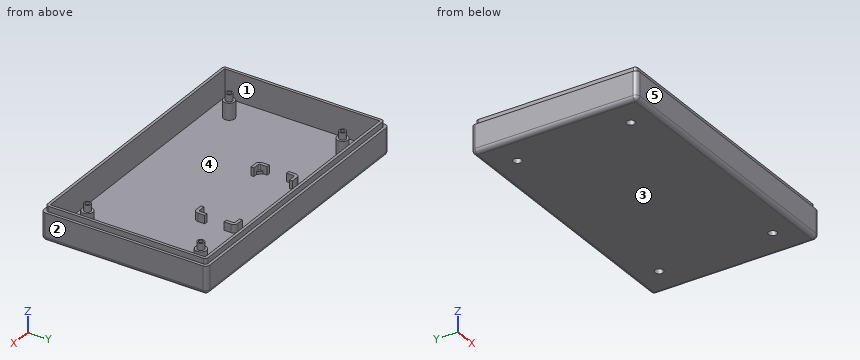
from build123d import *

# Parameters (mm, degrees)
SKETCH_1_W                  = 100
SKETCH_1_H                  = 60
EXTRUDE_1_DEPTH             = 2
SKETCH_2_W                  = 96
SKETCH_2_H                  = 56
EXTRUDE_2_DEPTH             = 10
SKETCH_3_W                  = 100
SKETCH_3_H                  = 60
SKETCH_3_W_2                = 98
SKETCH_3_H_2                = 58
CUT_EXTRUDE_1_DEPTH         = 2
EXTRUDE_3_DEPTH             = 3
EXTRUDE_4_DEPTH             = 1
FILLET_1_R                  = 0.5
FILLET_2_R                  = 1.5
SKETCH_6_R                  = 2
EXTRUDE_5_DEPTH             = 6
SKETCH_7_R                  = 1.2
EXTRUDE_6_DEPTH             = 2.5
SKETCH_8_R                  = 0.75
CUT_EXTRUDE_2_DEPTH         = 12.5
FILLET_3_R                  = 1.5
FILLET_4_R                  = 1.5
FILLET_5_R                  = 1
SKETCH_9_R                  = 1.5
CUT_EXTRUDE_3_DEPTH         = 7
PATTERN_LINEAR_1_COUNT      = 2
PATTERN_LINEAR_1_PITCH      = 78
PATTERN_LINEAR_1_COUNT_DIR2 = 2
PATTERN_LINEAR_1_PITCH_DIR2 = 41


with BuildPart() as part:
    # 草图1 → 凸台-拉伸1 (new body)
    with BuildSketch(Plane.XY):
        Rectangle(SKETCH_1_W, SKETCH_1_H)
    extrude(amount=EXTRUDE_1_DEPTH)

    # 草图2 → 凸台-拉伸2 (add)
    with BuildSketch(Plane.XY.offset(2)):
        Polygon((-47, 30), (-50, 30), (-50, 27), (-50, -27), (-50, -30), (-47, -30), (47, -30), (50, -30), (50, -27), (50, 27), (50, 30), (47, 30), align=None)
        Rectangle(SKETCH_2_W, SKETCH_2_H, mode=Mode.SUBTRACT)
    extrude(amount=EXTRUDE_2_DEPTH)

    # 草图3 → 切除-拉伸1 (cut)
    with BuildSketch(Plane.XY.offset(12)):
        Rectangle(SKETCH_3_W, SKETCH_3_H)
        Rectangle(SKETCH_3_W_2, SKETCH_3_H_2, mode=Mode.SUBTRACT)
    extrude(amount=-CUT_EXTRUDE_1_DEPTH, mode=Mode.SUBTRACT)

    # 草图4 → 凸台-拉伸3 (add)
    with BuildSketch(Plane.XY.offset(2)):
        Polygon((-16.61, 17.9), (-13.75, 17.9), (-13.75, 18.95), (-17.75, 18.95), (-17.75, 14.95), (-16.61, 14.95), align=None)
        Polygon((-16.61, 5), (-13.75, 5), (-13.75, 3.95), (-17.75, 3.95), (-17.75, 7.95), (-16.61, 7.95), align=None)
        Polygon((16.61, 17.9), (16.61, 14.95), (17.75, 14.95), (17.75, 18.95), (13.75, 18.95), (13.75, 17.9), align=None)
        Polygon((17.75, 3.95), (13.75, 3.95), (13.75, 5), (16.61, 5), (16.61, 7.95), (17.75, 7.95), align=None)
    extrude(amount=EXTRUDE_3_DEPTH)

    # 草图5 → 凸台-拉伸4 (add)
    with BuildSketch(Plane.XY.offset(2)):
        Polygon((-16.61, 17.9), (-15.11, 17.9), (-16.61, 16.4), align=None)
        Polygon((16.61, 17.9), (15.11, 17.9), (16.61, 16.4), align=None)
        Polygon((16.61, 5), (16.61, 6.5), (15.11, 5), align=None)
        Polygon((-16.61, 5), (-15.11, 5), (-16.61, 6.5), align=None)
    extrude(amount=EXTRUDE_4_DEPTH)

    # 圆角1
    fillet_1_edges = [part.edges().sort_by_distance(p)[0] for p in [
        (-16.61, 5, 4),
        (16.61, 17.9, 4),
        (-16.61, 17.9, 4),
        (16.61, 5, 4),
    ]]
    fillet(fillet_1_edges, radius=FILLET_1_R)

    # 圆角2
    fillet_2_edges = [part.edges().sort_by_distance(p)[0] for p in [
        (-17.75, 3.95, 3.5),
        (17.75, 18.95, 3.5),
        (-17.75, 18.95, 3.5),
        (17.75, 3.95, 3.5),
    ]]
    fillet(fillet_2_edges, radius=FILLET_2_R)

    # 草图6 → 凸台-拉伸5 (add)
    with BuildSketch(Plane.XY.offset(2)):
        with Locations((-39, 20.5)):
            Circle(SKETCH_6_R)
        with Locations((39, 20.5)):
            Circle(SKETCH_6_R)
        with Locations((39, -20.5)):
            Circle(SKETCH_6_R)
        with Locations((-39, -20.5)):
            Circle(SKETCH_6_R)
    extrude(amount=EXTRUDE_5_DEPTH)

    # 草图7 → 凸台-拉伸6 (add)
    with BuildSketch(Plane.XY.offset(8)):
        with Locations((-39, 20.5)):
            Circle(SKETCH_7_R)
        with Locations((39, 20.5)):
            Circle(SKETCH_7_R)
        with Locations((39, -20.5)):
            Circle(SKETCH_7_R)
        with Locations((-39, -20.5)):
            Circle(SKETCH_7_R)
    extrude(amount=EXTRUDE_6_DEPTH)

    # 草图8 → 切除-拉伸2 (cut)
    with BuildSketch(Plane.XY.offset(10.5)):
        with Locations((-39, 20.5)):
            Circle(SKETCH_8_R)
        with Locations((-39, -20.5)):
            Circle(SKETCH_8_R)
        with Locations((39, -20.5)):
            Circle(SKETCH_8_R)
        with Locations((39, 20.5)):
            Circle(SKETCH_8_R)
    extrude(amount=-CUT_EXTRUDE_2_DEPTH, mode=Mode.SUBTRACT)

    # 圆角3
    fillet_3_edges = [part.edges().sort_by_distance(p)[0] for p in [
        (-50, 30, 5),
        (50, 30, 5),
        (50, -30, 5),
        (-50, -30, 5),
    ]]
    fillet(fillet_3_edges, radius=FILLET_3_R)

    # 圆角4
    fillet_4_edges = [part.edges().sort_by_distance(p)[0] for p in [
        (0, 30, 0),
        (-50, 0, 0),
        (50, 0, 0),
        (0, -30, 0),
        (-49.560660172, 29.560660172, 0),
        (-49.560660172, -29.560660172, 0),
        (49.560660172, -29.560660172, 0),
        (49.560660172, 29.560660172, 0),
    ]]
    fillet(fillet_4_edges, radius=FILLET_4_R)

    # 圆角5
    fillet_5_edges = [part.edges().sort_by_distance(p)[0] for p in [
        (-49, 29, 11),
        (49, 29, 11),
        (49, -29, 11),
        (-49, -29, 11),
    ]]
    fillet(fillet_5_edges, radius=FILLET_5_R)

    # 草图9 → 切除-拉伸3 (cut)
    with BuildSketch(Plane(origin=(0, 0, 0), x_dir=(-1, 0, 0), z_dir=(0, 0, -1))):
        with Locations((-39, 20.5)):
            Circle(SKETCH_9_R)
    cut_extrude_3 = extrude(amount=-CUT_EXTRUDE_3_DEPTH, mode=Mode.SUBTRACT)

    # 阵列(线性)1: Cut-Extrude 3 2 × 2
    with Locations(*[(-i * PATTERN_LINEAR_1_PITCH, -j * PATTERN_LINEAR_1_PITCH_DIR2, 0) for i in range(PATTERN_LINEAR_1_COUNT) for j in range(PATTERN_LINEAR_1_COUNT_DIR2) if (i, j) != (0, 0)]):
        add(cut_extrude_3, mode=Mode.SUBTRACT)


solid = part.part
Geometry check sheet. Reference: the model listing, model coordinates, mm. Face numbers are marked on the shaded views. A direction names the side the tool comes from. Round coordinates to 2 decimals unless told otherwise and drop trailing zeros. Loops run counter-clockwise (first coordinate to the right, second up) from the corner with the lowest first, then second, coordinate; pieces in that order, holes last. Notation, with made-up numbers: (31, 84.25) -> (60, 84.25) arc R20 cw to (60, 93.25) -> close; hole circle Ø10 at (18, -18). An arc over 180 degrees is marked (long way). Answer as a JSON object with one key per item and string values. Group by question number.
Item 1: Release check for a two-part mould opening along Y. For the marked faces 3, 4 and 5 record: pulls with the +Y half, pulls with the -Y half, needs draft (parallel to the pull), parting line crosses it, or undercut.
Item 2: Set-up check for the marked faces 1 and 2: record each of +Z, -Z, +X, -X, +Y, -Y from which the full face is reachable in a straight line by a thin tool's end or side.
Item 3: Thickness scan on line 1 along Y through (x, z) = (-39, 9.3); line 2 along Y through (x, z) = (39, 3.75); line 3 along X through (y, z) = (25, 6.5). Record the ranges inside material, lowest first.
Item 4: Cross-section at A-A, the plane y = -2. Record the cut outline in (x, z).
Item 5: Cross-section at B-B, the plane x = -4.5. Record the cut outline in (y, z).
Item 6: Depth check by flat-ended pin: pin 1 Ø1.2 at (x, y) = (15.5, 17) entering from +Z; pin 2 Ø3 at (x, y) = (-39.5, -21) entering from +Z; pin 3 Ø1.6 at (x, y) = (16, 6) entering from +Z; pin 4 Ø12 at (x, y) = (-2, -16) entering from -Z. Enter the tip coordinate at first touch or a pass-through.
Determined:
{
 "1": {"face 3": "needs draft", "face 4": "undercut", "face 5": "pulls with the -Y half"},
 "2": {"face 1": "+Z", "face 2": "+Z, -Z, +X, +Y, -Y"},
 "3": {"line 1": "y = -30 to -28, -21.7 to -21.25, -19.75 to -19.3, 19.3 to 19.75, 21.25 to 21.7, 28 to 30", "line 2": "y = -30 to -28, -22.5 to -22, -19 to -18.5, 18.5 to 19, 22 to 22.5, 28 to 30", "line 3": "x = -50 to -48, 48 to 50"},
 "4": {"outline": "(-50, 1.5) arc R1.5 ccw to (-48.5, 0) -> (48.5, 0) arc R1.5 ccw to (50, 1.5) -> (50, 10) -> (49, 10) -> (49, 12) -> (48, 12) -> (48, 2) -> (-48, 2) -> (-48, 12) -> (-49, 12) -> (-49, 10) -> (-50, 10) -> close"},
 "5": {"outline": "(-30, 1.5) arc R1.5 ccw to (-28.5, 0) -> (28.5, 0) arc R1.5 ccw to (30, 1.5) -> (30, 10) -> (29, 10) -> (29, 12) -> (28, 12) -> (28, 2) -> (-28, 2) -> (-28, 12) -> (-29, 12) -> (-29, 10) -> (-30, 10) -> close"},
 "6": {"pin 1": "stops at z = 3", "pin 2": "stops at z = 10.5", "pin 3": "stops at z = 5", "pin 4": "stops at z = 0"}
}
